```python
from build123d import *

# Parameters (mm, degrees)
F0_R     = 5
F1_DEPTH = 20
F2_DEPTH = 800
F5_DEPTH = 10
F6_DEPTH = 10
F0_R_2   = 6
F7_DEPTH = 956


# Not quite as in the source:
# - a feature names something its author has since deleted; it is built from what else it names


with BuildPart() as f1:
    # F0 (on Top) → F1 (new body)
    with BuildSketch(Plane.XY):
        with BuildLine():
            ThreePointArc((-59.160797831, 10), (-42.4264068712, 42.4264068712), (-10, 59.160797831))
            Line((-10, 59.160797831), (-10, 60))
            Line((-10, 60), (-80, 60))
            Line((-80, 60), (-80, 10))
            Line((-80, 10), (-59.160797831, 10))
        make_face()
        with Locations((-70, 50)):
            Circle(F0_R, mode=Mode.SUBTRACT)
        with BuildLine():
            ThreePointArc((59.160797831, -10), (59.7898313673, -5.0175756168), (60, 0))
            ThreePointArc((60, 0), (59.7898313673, 5.0175756168), (59.160797831, 10))
            ThreePointArc((59.160797831, 10), (42.4264068712, 42.4264068712), (10, 59.160797831))
            ThreePointArc((10, 59.160797831), (5.0175756193, 59.7898313671), (5e-09, 60))
            ThreePointArc((5e-09, 60), (-5.0175756143, 59.7898313675), (-10, 59.160797831))
            ThreePointArc((-10, 59.160797831), (-42.4264068712, 42.4264068712), (-59.160797831, 10))
            ThreePointArc((-59.160797831, 10), (-60, 0), (-59.160797831, -10))
            ThreePointArc((-59.160797831, -10), (-42.4264068712, -42.4264068712), (-10, -59.160797831))
            ThreePointArc((-10, -59.160797831), (-5.0175756489, -59.7898313646), (-6.44e-08, -60))
            ThreePointArc((-6.44e-08, -60), (5.0175755847, -59.78983137), (10, -59.160797831))
            ThreePointArc((10, -59.160797831), (42.4264068712, -42.4264068712), (59.160797831, -10))
        make_face()
        with BuildLine():
            ThreePointArc((10, 59.160797831), (42.4264068712, 42.4264068712), (59.160797831, 10))
            Line((59.160797831, 10), (80, 10))
            Line((80, 10), (80, 60))
            Line((80, 60), (10, 60))
            Line((10, 60), (10, 59.160797831))
        make_face()
        with Locations((70, 50)):
            Circle(F0_R, mode=Mode.SUBTRACT)
        with BuildLine():
            ThreePointArc((59.160797831, 10), (59.7898313673, 5.0175756168), (60, 0))
            ThreePointArc((60, 0), (59.7898313673, -5.0175756168), (59.160797831, -10))
            Line((59.160797831, -10), (80, -10))
            Line((80, -10), (80, 10))
            Line((80, 10), (59.160797831, 10))
        make_face()
        with BuildLine():
            Line((80, -10), (59.160797831, -10))
            ThreePointArc((59.160797831, -10), (42.4264068712, -42.4264068712), (10, -59.160797831))
            Line((10, -59.160797831), (10, -60))
            Line((10, -60), (80, -60))
            Line((80, -60), (80, -10))
        make_face()
        with Locations((70, -50)):
            Circle(F0_R, mode=Mode.SUBTRACT)
        with BuildLine():
            ThreePointArc((-59.160797831, -10), (-60, 0), (-59.160797831, 10))
            Line((-59.160797831, 10), (-80, 10))
            Line((-80, 10), (-80, -10))
            Line((-80, -10), (-59.160797831, -10))
        make_face()
        with BuildLine():
            Line((-10, -60), (-10, -59.160797831))
            ThreePointArc((-10, -59.160797831), (-42.4264068712, -42.4264068712), (-59.160797831, -10))
            Line((-59.160797831, -10), (-80, -10))
            Line((-80, -10), (-80, -60))
            Line((-80, -60), (-10, -60))
        make_face()
        with Locations((-70, -50)):
            Circle(F0_R, mode=Mode.SUBTRACT)
        with BuildLine():
            Line((-10, -60), (-6.44e-08, -60))
            ThreePointArc((-6.44e-08, -60), (-5.0175756489, -59.7898313646), (-10, -59.160797831))
            Line((-10, -59.160797831), (-10, -60))
        make_face()
        with BuildLine():
            Line((10, -60), (10, -59.160797831))
            ThreePointArc((10, -59.160797831), (5.0175755847, -59.78983137), (-6.44e-08, -60))
            Line((-6.44e-08, -60), (10, -60))
        make_face()
        with BuildLine():
            ThreePointArc((-10, 59.160797831), (-5.0175756143, 59.7898313675), (5e-09, 60))
            Line((5e-09, 60), (-10, 60))
            Line((-10, 60), (-10, 59.160797831))
        make_face()
        with BuildLine():
            ThreePointArc((5e-09, 60), (5.0175756193, 59.7898313671), (10, 59.160797831))
            Line((10, 59.160797831), (10, 60))
            Line((10, 60), (5e-09, 60))
        make_face()
    extrude(amount=F1_DEPTH)

    # F0 (on Top) → F2 (join)
    with BuildSketch(Plane.XY):
        with BuildLine():
            ThreePointArc((59.160797831, -10), (59.7898313673, -5.0175756168), (60, 0))
            ThreePointArc((60, 0), (59.7898313673, 5.0175756168), (59.160797831, 10))
            ThreePointArc((59.160797831, 10), (42.4264068712, 42.4264068712), (10, 59.160797831))
            ThreePointArc((10, 59.160797831), (5.0175756193, 59.7898313671), (5e-09, 60))
            ThreePointArc((5e-09, 60), (-5.0175756143, 59.7898313675), (-10, 59.160797831))
            ThreePointArc((-10, 59.160797831), (-42.4264068712, 42.4264068712), (-59.160797831, 10))
            ThreePointArc((-59.160797831, 10), (-60, 0), (-59.160797831, -10))
            ThreePointArc((-59.160797831, -10), (-42.4264068712, -42.4264068712), (-10, -59.160797831))
            ThreePointArc((-10, -59.160797831), (-5.0175756489, -59.7898313646), (-6.44e-08, -60))
            ThreePointArc((-6.44e-08, -60), (5.0175755847, -59.78983137), (10, -59.160797831))
            ThreePointArc((10, -59.160797831), (42.4264068712, -42.4264068712), (59.160797831, -10))
        make_face()
    extrude(amount=-F2_DEPTH)

    # F4 (on Right) → F5 (join, symmetric)
    with BuildSketch(Plane.YZ):
        Polygon((95, -760), (0, -760), (-95, -760), (-95, -780), (95, -780), align=None)
    extrude(amount=F5_DEPTH, both=True)

    # F3 (on Front) → F6 (join, symmetric)
    with BuildSketch(Plane.XZ):
        Polygon((102.5, -760), (0, -760), (-102.5, -760), (-102.5, -780), (102.5, -780), align=None)
    extrude(amount=F6_DEPTH, both=True)

    # F0 (on Top) → F7 (cut)
    with BuildSketch(Plane.XY):
        with Locations((0, 80)):
            Circle(F0_R_2)
        with Locations((0, -80)):
            Circle(F0_R_2)
        with Locations((87.5, 0)):
            Circle(F0_R_2)
        with Locations((-87.5, 0)):
            Circle(F0_R_2)
    extrude(amount=-F7_DEPTH, mode=Mode.SUBTRACT)


solid = f1.part
```
Input: part model. Units: mm. Frame: model coordinates. A direction names the side the tool comes from. Coordinates: 2 decimals unless noted, no trailing zeros. Write each loop counter-clockwise with the first axis right and the second up, starting at its lowest first coordinate (ties: lowest second). Pieces come first, ordered by that corner, then holes. Notation, with made-up numbers: (63.25, -35.75) - (93.25, -35.75) arc R35 cw to (93.25, 1.25) - close; hole circle Ø11 at (14.5, 39). An arc over 180 degrees is marked (long way). Put each result on its own line as item: value. Start each with the question number.
1) Cut plane C-C (y = 34.5). Return the cut outline in (x, z).
2) Cut plane A-A (z = -144). Return the cut outline in (x, y), plus the area to 3 significant figures.
3) Cut plane B-B (x = -41.5). Return the cut outline in (y, z).
4) Contact query for flat-ended pins moving along their axis: pin 1 (5 mm diameter, centred on y = 58, z = -430.5, fed in from -X); pin 2 (16 mm diameter, centred on x = -78.5, z = -766.5, fed in from +Y); pin 3 (4 mm diameter, centred on x = 17.5, z = -496, fed in from +Y); pin 4 (9 mm diameter, centred on x = 70, y = -50, fed in from +Z). Output: stop coordinate, or through.
5) Reachability of faces 4 (the face through (81, -10, -770)), 5 (the face through (0, -95, -770)), 6 (the face through (-81, -10, -770)), 7 (the face through (81, 10, -770)) from +Z, -Z, +X, -X, +Y, -Y: full face, straight path, thin tool, end or side. Return the list, or none.
6) Ray query, L1, parallel to Y at x = -70, z = 5.5; L2, parallel to Y at x = 0, z = -768.75; L3, parallel to Z at x = -8, y = -70.5. Return the intervals inside material, ascending.
7) Mould query, pull axis Z, two halves, no side actions, for faces 1 (the face through (81, 0, -760)), 2 (the face through (-1, -60, 10)), 3 (the face through (-1, 1, -800)). Classes: pulls with the +Z half, pulls with the -Z half, needs draft (parallel to the pull), parting line crosses it, or undercut.
Resolved:
1. outline: (-80, 0) - (-49.09, 0) - (-49.09, -800) - (49.09, -800) - (49.09, 0) - (80, 0) - (80, 20) - (-80, 20) - close
2. outline: circle Ø120 at (0, 0)
2. area: 11,300 mm2
3. outline: (-60, 0) - (-43.33, 0) - (-43.33, -800) - (43.33, -800) - (43.33, 0) - (60, 0) - (60, 20) - (-60, 20) - close
4. pin 1: stops at x = -22.8
4. pin 2: stops at y = 10
4. pin 3: stops at y = 57.96
4. pin 4: passes through
5. face 4: -Z, +X, -Y
5. face 5: +Z, -Z, +X, -X, -Y
5. face 6: -Z, -X, -Y
5. face 7: -Z, +X, +Y
6. L1: y = -60 to -55, -45 to 45, 55 to 60
6. L2: y = -95 to -86, -74 to 74, 86 to 95
6. L3: z = -780 to -760
7. face 1: undercut
7. face 2: needs draft
7. face 3: pulls with the -Z half
